from build123d import *

# Parameters (mm, degrees)
SKETCH1_W               = 170
SKETCH1_H               = 28
BOSS_EXTRUDE1_DEPTH     = 1.5
SKETCH2_W               = 28
SKETCH2_H               = 85
BOSS_EXTRUDE2_DEPTH     = 1.5
FILLET2_R               = 10
FILLET3_R               = 1
FILLET4_R               = 1
SKETCH5_R               = 1.5
CUT_EXTRUDE2_DEPTH      = 15
CUT_EXTRUDE2_DEPTH_BACK = 15
SKETCH7_R               = 3.5
CUT_EXTRUDE3_DEPTH      = 15
CUT_EXTRUDE3_DEPTH_BACK = 15
SKETCH8_R               = 1.5
CUT_EXTRUDE4_DEPTH      = 15
CUT_EXTRUDE4_DEPTH_BACK = 15
SKETCH11_W              = 28
SKETCH11_H              = 85
SKETCH11_R              = 1
BOSS_EXTRUDE5_DEPTH     = 1.5
FILLET5_R               = 1
FILLET6_R               = 1
FILLET7_R               = 10
FILLET8_R               = 10
SKETCH12_R              = 1.5
CUT_EXTRUDE5_DEPTH      = 10
CUT_EXTRUDE5_DEPTH_BACK = 10
SKETCH13_R              = 1.5
CUT_EXTRUDE6_DEPTH      = 10
CUT_EXTRUDE6_DEPTH_BACK = 10


with BuildPart() as part:
    # Sketch1 → Boss-Extrude1 (new body)
    with BuildSketch(Plane(origin=(0, 0, 0), x_dir=(1, 0, 0), z_dir=(0, 1, 0))):
        with Locations((85, 14)):
            Rectangle(SKETCH1_W, SKETCH1_H)
    extrude(amount=BOSS_EXTRUDE1_DEPTH)

    # Sketch2 → Boss-Extrude2 (add)
    with BuildSketch(Plane(origin=(0, 0, 0), x_dir=(0, 0, -1), z_dir=(1, 0, 0))):
        with Locations((14, 42.5)):
            Rectangle(SKETCH2_W, SKETCH2_H)
    extrude(amount=-BOSS_EXTRUDE2_DEPTH)

    # Fillet2
    fillet2_edges = [part.edges().sort_by_distance(p)[0] for p in [
        (-0.75, 85, -28),
        (-0.75, 85, 0),
    ]]
    fillet(fillet2_edges, radius=FILLET2_R)

    # Fillet3
    fillet3_edges = [part.edges().sort_by_distance(p)[0] for p in [
        (-1.5, 0, -14),
    ]]
    fillet(fillet3_edges, radius=FILLET3_R)

    # Fillet4
    fillet4_edges = [part.edges().sort_by_distance(p)[0] for p in [
        (0, 1.5, -14),
    ]]
    fillet(fillet4_edges, radius=FILLET4_R)

    # Sketch5 → Cut-Extrude2 (cut, two sides)
    with BuildSketch(Plane(origin=(0, 0, 0), x_dir=(0, 0, -1), z_dir=(1, 0, 0))) as cut_extrude2_sk:
        with Locations((14, 77)):
            Circle(SKETCH5_R)
        with Locations((14, 60)):
            Circle(SKETCH5_R)
        with Locations((22.5, 68.5)):
            Circle(SKETCH5_R)
        with Locations((5.5, 68.5)):
            Circle(SKETCH5_R)
    extrude(amount=CUT_EXTRUDE2_DEPTH, mode=Mode.SUBTRACT)
    extrude(cut_extrude2_sk.sketch, amount=-CUT_EXTRUDE2_DEPTH_BACK, mode=Mode.SUBTRACT)

    # Sketch7 → Cut-Extrude3 (cut, two sides)
    with BuildSketch(Plane(origin=(0, 0, 0), x_dir=(0, 0, -1), z_dir=(1, 0, 0))) as cut_extrude3_sk:
        with Locations((14, 37.5)):
            Circle(SKETCH7_R)
    extrude(amount=CUT_EXTRUDE3_DEPTH, mode=Mode.SUBTRACT)
    extrude(cut_extrude3_sk.sketch, amount=-CUT_EXTRUDE3_DEPTH_BACK, mode=Mode.SUBTRACT)

    # Sketch8 → Cut-Extrude4 (cut, two sides)
    with BuildSketch(Plane(origin=(0, 1.5, 0), x_dir=(1, 0, 0), z_dir=(0, 1, 0))) as cut_extrude4_sk:
        with Locations((161, 7)):
            Circle(SKETCH8_R)
        with Locations((11, 21)):
            Circle(SKETCH8_R)
        with Locations((11, 7)):
            Circle(SKETCH8_R)
        with Locations((161, 21)):
            Circle(SKETCH8_R)
    extrude(amount=CUT_EXTRUDE4_DEPTH, mode=Mode.SUBTRACT)
    extrude(cut_extrude4_sk.sketch, amount=-CUT_EXTRUDE4_DEPTH_BACK, mode=Mode.SUBTRACT)

    # Sketch11 → Boss-Extrude5 (add)
    with BuildSketch(Plane(origin=(170, 0, 0), x_dir=(0, 0, -1), z_dir=(1, 0, 0))):
        with Locations((14, 42.5)):
            Rectangle(SKETCH11_W, SKETCH11_H)
        with Locations((14, 67.5)):
            Circle(SKETCH11_R, mode=Mode.SUBTRACT)
    extrude(amount=BOSS_EXTRUDE5_DEPTH)

    # Fillet5
    fillet5_edges = [part.edges().sort_by_distance(p)[0] for p in [
        (170, 1.5, -14),
    ]]
    fillet(fillet5_edges, radius=FILLET5_R)

    # Fillet6
    fillet6_edges = [part.edges().sort_by_distance(p)[0] for p in [
        (171.5, 0, -14),
    ]]
    fillet(fillet6_edges, radius=FILLET6_R)

    # Fillet7
    fillet7_edges = [part.edges().sort_by_distance(p)[0] for p in [
        (170.75, 85, 0),
    ]]
    fillet(fillet7_edges, radius=FILLET7_R)

    # Fillet8
    fillet8_edges = [part.edges().sort_by_distance(p)[0] for p in [
        (170.75, 85, -28),
    ]]
    fillet(fillet8_edges, radius=FILLET8_R)

    # Sketch12 → Cut-Extrude5 (cut, two sides)
    with BuildSketch(Plane.ZY.offset(-170)) as cut_extrude5_sk:
        with Locations((-21, 79.5)):
            Circle(SKETCH12_R)
        with Locations((-7, 79.5)):
            Circle(SKETCH12_R)
        with Locations((-7, 55.5)):
            Circle(SKETCH12_R)
        with Locations((-21, 55.5)):
            Circle(SKETCH12_R)
    extrude(amount=CUT_EXTRUDE5_DEPTH, mode=Mode.SUBTRACT)
    extrude(cut_extrude5_sk.sketch, amount=-CUT_EXTRUDE5_DEPTH_BACK, mode=Mode.SUBTRACT)

    # Sketch13 → Cut-Extrude6 (cut, two sides)
    with BuildSketch(Plane(origin=(0, 1.5, 0), x_dir=(1, 0, 0), z_dir=(0, 1, 0))) as cut_extrude6_sk:
        with Locations((85, 22.5)):
            Circle(SKETCH13_R)
        with Locations((85, 5.5)):
            Circle(SKETCH13_R)
        with Locations((93.5, 14)):
            Circle(SKETCH13_R)
        with Locations((76.5, 14)):
            Circle(SKETCH13_R)
    extrude(amount=CUT_EXTRUDE6_DEPTH, mode=Mode.SUBTRACT)
    extrude(cut_extrude6_sk.sketch, amount=-CUT_EXTRUDE6_DEPTH_BACK, mode=Mode.SUBTRACT)


solid = part.part
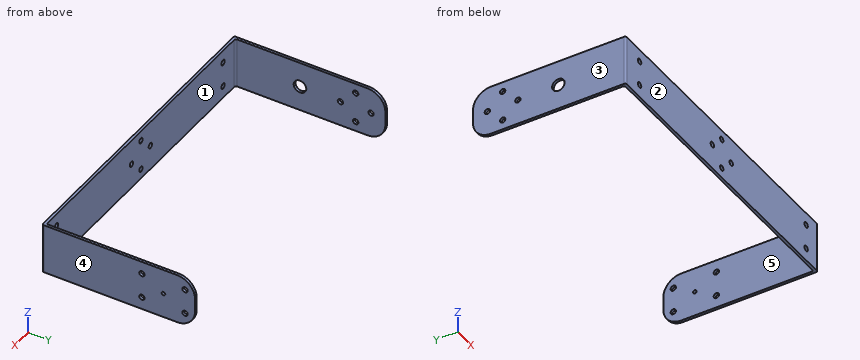
CAD build for the part. Positions are in the model's coordinates, mm. Face numbers are marked on the shaded views. A direction names the side the tool comes from. Round coordinates to 2 decimals unless told otherwise and drop trailing zeros. Loops run counter-clockwise (first coordinate to the right, second up) from the corner with the lowest first, then second, coordinate; pieces in that order, holes last.
(1) Cut at C-C (x = 99). Give the cut face in (y, z), plus the area to 3 significant figures.
(2) Wall check: line 1 along Z through (x, y) = (76.5, 0.95); line 2 along X through (y, z) = (19.5, -24); line 3 along Y through (x, z) = (55.5, -19.5). Give the ranges that are in metal, low to high.
(3) Two-plate mould, pull along X, no slides. Class the marked faces 1, 2 and 3: +X half, -X half, draft (parallel to the pull), parting line (faces both ways), or undercut.
(4) Which spindle directions (+Z, -Z, +X, -X, +Y, -Y) get a long thin tool onto all of the face, cutting with end or side? Do the marked faces 4 and 5. Say none if no direction does.
(5) Drop flat-ended pins along their axis: pin 1 (12 mm diameter, centred on x = 153, z = -21, fed in from -Y); pin 2 (1.8 mm diameter, centred on y = 79.5, z = -21, fed in from +X); pin 3 (2.5 mm diameter, centred on x = 11, z = -7, fed in from +Y); pin 4 (2.5 mm diameter, centred on y = 77, z = -14, fed in from -X). Give the stop position or say it passes through.
(6) Cut at A-A (y = 46). Give the cut face in (x, z), plus the area to 3 significant figures.
(7) Cut at B-B (y = 37.5). Give the cut face in (x, z).
Findings below:
1. outline: (0, -28) - (1.5, -28) - (1.5, 0) - (0, 0) - close
1. area: 42.0 mm2
2. line 1: z = -28 to -15.5, -12.5 to 0
2. line 2: x = -1.5 to 0, 170 to 171.5
2. line 3: y = 0 to 1.5
3. face 1: undercut
3. face 2: draft
3. face 3: -X half
4. face 4: +Z, -Z, +X, +Y, -Y
4. face 5: +Z, -Z, +Y
5. pin 1: stops at y = 0
5. pin 2: stops at x = 0
5. pin 3: passes through
5. pin 4: stops at x = 170
6. outline: (-1.5, -28) - (0, -28) - (0, 0) - (-1.5, 0) - close; (170, -28) - (171.5, -28) - (171.5, 0) - (170, 0) - close
6. area: 84.0 mm2
7. outline: (-1.5, -28) - (0, -28) - (0, -17.5) - (-1.5, -17.5) - close; (-1.5, -10.5) - (0, -10.5) - (0, 0) - (-1.5, 0) - close; (170, -28) - (171.5, -28) - (171.5, 0) - (170, 0) - close
